CAD build for the part. Positions are in the model's coordinates, mm. Face numbers are marked on the shaded views. A direction names the side the tool comes from. Round coordinates to 2 decimals unless told otherwise and drop trailing zeros. Loops run counter-clockwise (first coordinate to the right, second up) from the corner with the lowest first, then second, coordinate; pieces in that order, holes last. Notation, with made-up numbers: (19, -27.5) -> (47, -27.5) arc R32 cw to (47, 6.5) -> close; hole circle Ø3 at (47.5, 40). An arc over 180 degrees is marked (long way). Answer as CSV lines item,"result".
```python
from build123d import *

# Parameters (mm, degrees)
F0_R     = 31.716166
F1_DEPTH = 53.594
F2_R     = 5.08
F3_W     = 40.479297
F3_H     = 50.922095
F4_DEPTH = 132.588


with BuildPart() as f1:
    # F0 (on Top) → F1 (new body)
    with BuildSketch(Plane.XY):
        Circle(F0_R)
    extrude(amount=F1_DEPTH)

    # F2
    f2_edges = [f1.edges().sort_by_distance(p)[0] for p in [
        (-31.716166, 0, 53.594),
        (-31.716166, 0, 0),
    ]]
    fillet(f2_edges, radius=F2_R)

    # F3 (on Top) → F4 (cut)
    with BuildSketch(Plane.XY):
        with Locations((-45.781928, -11.702132)):
            Rectangle(F3_W, F3_H)
    extrude(amount=F4_DEPTH, mode=Mode.SUBTRACT)


solid = f1.part
```
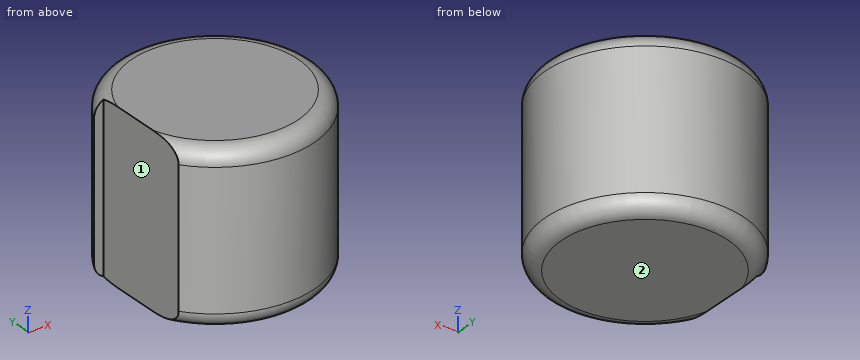
Q1. Tool access for the marked faces 1 and 2: list every direction of +Z, -Z, +X, -X, +Y, -Y with a clear straight run to the whole face (end or side of a thin tool).
Results:
face 1,"+Z, -Z, -X, -Y"
face 2,"-Z, +X, -X, +Y, -Y"
Q2. Probe L1, parallel to Z at x = -14, y = -23; L2, parallel to X at y = -0.5, z = 31.5; L3, parallel to X at y = -14, z = 22. List the from-to ranges inside material, lowest first. Write a range as [from, to].
Results:
L1,"[0.01, 53.59]"
L2,"[-25.54, 31.71]"
L3,"[-25.54, 28.46]"
Q3. Slice it at A-A, the plane y = 0. Give the cut face in (x, z).
Results:
outline,"(-25.54, 0) -> (26.64, 0) arc R5.08 ccw to (31.72, 5.08) -> (31.72, 48.51) arc R5.08 ccw to (26.64, 53.59) -> (-25.54, 53.59) -> close"
Q4. Slice it at B-B, the plane z = 40. Give the cut face in (x, y).
Results:
outline,"(-28.58, 13.76) -> (-25.54, 13.76) -> (-25.54, -18.8) arc R31.72 ccw (long way) to start"
Q5. Drop flat-ended pins along their axis: pin 1 Ø8 at (x, z) = (21, 33.5) entering from -Y; pin 2 Ø1.5 at (x, z) = (16.5, 37) entering from -Y; pin 3 Ø2.5 at (x, z) = (-27, 32) entering from -Y; pin 4 Ø4 at (x, y) = (21.5, 15.5) entering from -Z. Give the stop position or say it passes through.
Results:
pin 1,"y = -26.78"
pin 2,"y = -27.53"
pin 3,"y = 13.76"
pin 4,"z = 0"
